```python
from build123d import *

# Parameters (mm, degrees)
DODANIE_WYCI_GNI_CIE1_DEPTH = 85


with BuildPart() as part:
    # Szkic1 → Dodanie-wyciągnięcie1 (new body)
    with BuildSketch(Plane(origin=(0, 0, 0), x_dir=(1, 0, 0), z_dir=(0, 1, 0))):
        with BuildLine():
            Line((0, 3.9), (2.839339828, 3.9))
            Line((2.839339828, 3.9), (5.5, 6.560660172))
            Line((5.5, 6.560660172), (5.5, 8.2))
            Line((5.5, 8.2), (3.1, 8.2))
            Line((3.1, 8.2), (3.1, 10))
            Line((3.1, 10), (8.5, 10))
            ThreePointArc((8.5, 10), (9.560660172, 9.560660172), (10, 8.5))
            Line((10, 8.5), (10, 3.1))
            Line((10, 3.1), (8.2, 3.1))
            Line((8.2, 3.1), (8.2, 5.5))
            Line((8.2, 5.5), (6.560660172, 5.5))
            Line((6.560660172, 5.5), (3.9, 2.839339828))
            Line((3.9, 2.839339828), (3.9, 0))
            Line((3.9, 0), (3.9, -2.839339828))
            Line((3.9, -2.839339828), (6.560660172, -5.5))
            Line((6.560660172, -5.5), (8.2, -5.5))
            Line((8.2, -5.5), (8.2, -3.1))
            Line((8.2, -3.1), (10, -3.1))
            Line((10, -3.1), (10, -8.5))
            ThreePointArc((10, -8.5), (9.560660172, -9.560660172), (8.5, -10))
            Line((8.5, -10), (3.1, -10))
            Line((3.1, -10), (3.1, -8.2))
            Line((3.1, -8.2), (5.5, -8.2))
            Line((5.5, -8.2), (5.5, -6.560660172))
            Line((5.5, -6.560660172), (2.839339828, -3.9))
            Line((2.839339828, -3.9), (0, -3.9))
            Line((0, -3.9), (-2.839339828, -3.9))
            Line((-2.839339828, -3.9), (-5.5, -6.560660172))
            Line((-5.5, -6.560660172), (-5.5, -8.2))
            Line((-5.5, -8.2), (-3.1, -8.2))
            Line((-3.1, -8.2), (-3.1, -10))
            Line((-3.1, -10), (-8.5, -10))
            ThreePointArc((-8.5, -10), (-9.560660172, -9.560660172), (-10, -8.5))
            Line((-10, -8.5), (-10, -3.1))
            Line((-10, -3.1), (-8.2, -3.1))
            Line((-8.2, -3.1), (-8.2, -5.5))
            Line((-8.2, -5.5), (-6.560660172, -5.5))
            Line((-6.560660172, -5.5), (-3.9, -2.839339828))
            Line((-3.9, -2.839339828), (-3.9, 0))
            Line((-3.9, 0), (-3.9, 2.839339828))
            Line((-3.9, 2.839339828), (-6.560660172, 5.5))
            Line((-6.560660172, 5.5), (-8.2, 5.5))
            Line((-8.2, 5.5), (-8.2, 3.1))
            Line((-8.2, 3.1), (-10, 3.1))
            Line((-10, 3.1), (-10, 8.5))
            ThreePointArc((-10, 8.5), (-9.560660172, 9.560660172), (-8.5, 10))
            Line((-8.5, 10), (-3.1, 10))
            Line((-3.1, 10), (-3.1, 8.2))
            Line((-3.1, 8.2), (-5.5, 8.2))
            Line((-5.5, 8.2), (-5.5, 6.560660172))
            Line((-5.5, 6.560660172), (-2.839339828, 3.9))
            Line((-2.839339828, 3.9), (0, 3.9))
        make_face()
        with BuildLine():
            ThreePointArc((2.5, 0), (1.767766953, 1.767766953), (0, 2.5))
            ThreePointArc((0, 2.5), (-1.767766953, 1.767766953), (-2.5, 0))
            ThreePointArc((-2.5, 0), (-1.767766953, -1.767766953), (0, -2.5))
            ThreePointArc((0, -2.5), (1.767766953, -1.767766953), (2.5, 0))
        make_face(mode=Mode.SUBTRACT)
    extrude(amount=DODANIE_WYCI_GNI_CIE1_DEPTH)


solid = part.part
```
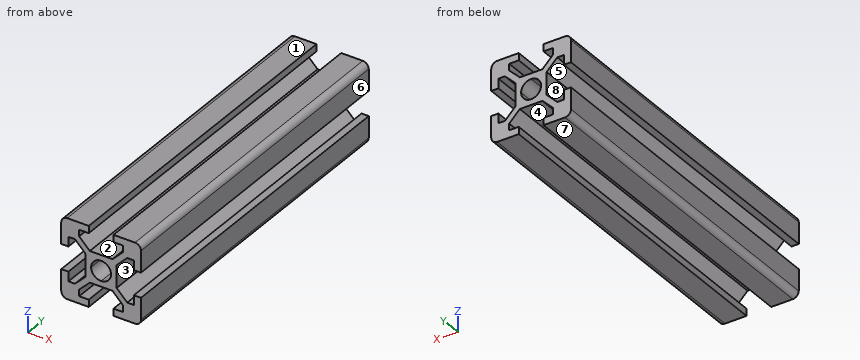
Build history of the part. All positions in model axes, mm. Face numbers are marked on the shaded views. A direction names the side the tool comes from. Coordinates: 2 decimals unless noted, no trailing zeros. Order: outer loops, then holes, each group sorted by start corner. A loop starts at its lowest first (then second) coordinate and runs counter-clockwise, first axis right, second up. Notation, with made-up numbers: (-26.5, -9) -> (24.5, -9) arc R26 cw to (24.5, 18) -> close; hole circle Ø10 at (60, 6). An arc over 180 degrees is marked (long way). Answer in a Markdown table with one row per item. Add a question column.
Q1. Band-saw the part on B-B, the plane x = -1.25. List the corners of the cut face in (y, z).
Q2. Band-saw the part on A-A, the plane z = 1.75. List the corners of the cut face in (x, y), then the cut area to 3 significant figures.
Q3. Drop flat-ended pins along their axis: pin 1 (1.4 mm diameter, centred on y = 55, z = -9.5, fed in from +X); pin 2 (1.4 mm diameter, centred on x = -9.5, y = 29, fed in from +Z); pin 3 (1.4 mm diameter, centred on x = 9.5, y = 52, fed in from -Z). Give the stop position or say it passes through.
Q4. Wall check: line 1 along Z through (x, y) = (-7.75, 72); line 2 along Z through (x, y) = (-4, 31). Give the ranges that are in metal, low to high. Write a range as [from, to].
Q5. Which spindle directions (+Z, -Z, +X, -X, +Y, -Y) get a long thin tool onto all of the face, cutting with end or side? Do the marked faces 4, 5, 6, 7 and 8. Say none if no direction does.
Q6. Mould opens along X. For the marked faces 1, 2 and 3 say: +X half, -X half, draft (parallel to the pull), parting line (faces both ways), or undercut.
Answers follow:
| question | item | result |
|---|---|---|
| 1 | outline | (0, -3.9) -> (85, -3.9) -> (85, -2.17) -> (0, -2.17) -> close; (0, 2.17) -> (85, 2.17) -> (85, 3.9) -> (0, 3.9) -> close |
| 2 | outline | (-3.9, 0) -> (-1.79, 0) -> (-1.79, 85) -> (-3.9, 85) -> close; (1.79, 0) -> (3.9, 0) -> (3.9, 85) -> (1.79, 85) -> close |
| 2 | area | 359 mm^2 |
| 3 | pin 1 | x = 9.97 |
| 3 | pin 2 | z = 9.97 |
| 3 | pin 3 | z = -9.97 |
| 4 | line 1 | [-10, -5.5], [5.5, 10] |
| 4 | line 2 | [-10, -8.2], [-5.06, -2.94], [2.94, 5.06], [8.2, 10] |
| 5 | face 4 | -Z, +Y, -Y |
| 5 | face 5 | +Y, -Y |
| 5 | face 6 | +Z, -Z, +X, +Y, -Y |
| 5 | face 7 | -Z, +X, -X, +Y, -Y |
| 5 | face 8 | -X, +Y, -Y |
| 6 | face 1 | draft |
| 6 | face 2 | undercut |
| 6 | face 3 | +X half |
